from build123d import *

# Parameters (mm, degrees)
BOSS_EXTRUDE1_DEPTH                                 = 15
M24X2_0_TAPPED_HOLE1_D                              = 22
M24X2_0_TAPPED_HOLE1_DEPTH                          = 58
M24X2_0_TAPPED_HOLE1_TIP                            = 6.609466809
CBORE_FOR_M5_HEX_SOCKET_HEAD_CAP_SCREW1_D           = 5.5
CBORE_FOR_M5_HEX_SOCKET_HEAD_CAP_SCREW1_CBORE_D     = 8.5
CBORE_FOR_M5_HEX_SOCKET_HEAD_CAP_SCREW1_CBORE_DEPTH = 5
CIRPATTERN3_COUNT                                   = 6


with BuildPart() as part:
    # Sketch1 → Boss-Extrude1 (new body)
    with BuildSketch(Plane.XY):
        with BuildLine():
            Line((-2.5, 29), (2.5, 29))
            Line((2.5, 29), (2.991048754, 29.850521392))
            ThreePointArc((2.991048754, 29.850521392), (9.270509831, 28.531695489), (15.125886974, 25.907673443))
            Line((15.125886974, 25.907673443), (15.023229831, 24.930955968))
            Line((15.023229831, 24.930955968), (19.068314802, 21.992029706))
            Line((19.068314802, 21.992029706), (19.965505521, 22.39148475))
            ThreePointArc((19.965505521, 22.39148475), (24.270509831, 17.633557569), (27.465247988, 12.068974809))
            Line((27.465247988, 12.068974809), (26.808096487, 11.339134128))
            Line((26.808096487, 11.339134128), (28.353181458, 6.583851546))
            Line((28.353181458, 6.583851546), (29.31381778, 6.379661993))
            ThreePointArc((29.31381778, 6.379661993), (30, 0), (29.31381778, -6.379661993))
            Line((29.31381778, -6.379661993), (28.353181458, -6.583851546))
            Line((28.353181458, -6.583851546), (26.808096487, -11.339134128))
            Line((26.808096487, -11.339134128), (27.465247988, -12.068974809))
            ThreePointArc((27.465247988, -12.068974809), (24.270509831, -17.633557569), (19.965505521, -22.39148475))
            Line((19.965505521, -22.39148475), (19.068314802, -21.992029706))
            Line((19.068314802, -21.992029706), (15.023229831, -24.930955968))
            Line((15.023229831, -24.930955968), (15.125886974, -25.907673443))
            ThreePointArc((15.125886974, -25.907673443), (9.270509831, -28.531695489), (2.991048754, -29.850521392))
            Line((2.991048754, -29.850521392), (2.5, -29))
            Line((2.5, -29), (-2.5, -29))
            Line((-2.5, -29), (-2.991048754, -29.850521392))
            ThreePointArc((-2.991048754, -29.850521392), (-9.270509831, -28.531695489), (-15.125886974, -25.907673443))
            Line((-15.125886974, -25.907673443), (-15.023229831, -24.930955968))
            Line((-15.023229831, -24.930955968), (-19.068314802, -21.992029706))
            Line((-19.068314802, -21.992029706), (-19.965505521, -22.39148475))
            ThreePointArc((-19.965505521, -22.39148475), (-24.270509831, -17.633557569), (-27.465247988, -12.068974809))
            Line((-27.465247988, -12.068974809), (-26.808096487, -11.339134128))
            Line((-26.808096487, -11.339134128), (-28.353181458, -6.583851546))
            Line((-28.353181458, -6.583851546), (-29.31381778, -6.379661993))
            ThreePointArc((-29.31381778, -6.379661993), (-30, 0), (-29.31381778, 6.379661993))
            Line((-29.31381778, 6.379661993), (-28.353181458, 6.583851546))
            Line((-28.353181458, 6.583851546), (-26.808096487, 11.339134128))
            Line((-26.808096487, 11.339134128), (-27.465247988, 12.068974809))
            ThreePointArc((-27.465247988, 12.068974809), (-24.270509831, 17.633557569), (-19.965505521, 22.39148475))
            Line((-19.965505521, 22.39148475), (-19.068314802, 21.992029706))
            Line((-19.068314802, 21.992029706), (-15.023229831, 24.930955968))
            Line((-15.023229831, 24.930955968), (-15.125886974, 25.907673443))
            ThreePointArc((-15.125886974, 25.907673443), (-9.270509831, 28.531695489), (-2.991048754, 29.850521392))
            Line((-2.991048754, 29.850521392), (-2.5, 29))
        make_face()
    extrude(amount=BOSS_EXTRUDE1_DEPTH)

    # M24x2.0 Tapped Hole1
    with Locations(Plane.XY.offset(15)):
        with Locations((0, 0)):
            Hole(M24X2_0_TAPPED_HOLE1_D / 2, depth=M24X2_0_TAPPED_HOLE1_DEPTH)
            with Locations((0, 0, -(M24X2_0_TAPPED_HOLE1_DEPTH + M24X2_0_TAPPED_HOLE1_TIP / 2))):  # 118° drill point
                Cone(0, M24X2_0_TAPPED_HOLE1_D / 2, M24X2_0_TAPPED_HOLE1_TIP, mode=Mode.SUBTRACT)

    # CBORE for M5 Hex Socket Head Cap Screw1 (through all)
    with Locations(Plane.XY.offset(15)):
        with Locations((0, 19)):
            cbore_for_m5_hex_socket_head_cap_screw1 = CounterBoreHole(CBORE_FOR_M5_HEX_SOCKET_HEAD_CAP_SCREW1_D / 2, CBORE_FOR_M5_HEX_SOCKET_HEAD_CAP_SCREW1_CBORE_D / 2, CBORE_FOR_M5_HEX_SOCKET_HEAD_CAP_SCREW1_CBORE_DEPTH)

    # CirPattern3: CBORE for M5 Hex Socket Head Cap Screw1 ×6 about axis
    cirpattern3_axis = Axis((0, 0, 0), (0, 0, 1))
    for i in range(1, CIRPATTERN3_COUNT):
        add(cbore_for_m5_hex_socket_head_cap_screw1.rotate(cirpattern3_axis, i * 360 / CIRPATTERN3_COUNT), mode=Mode.SUBTRACT)


solid = part.part
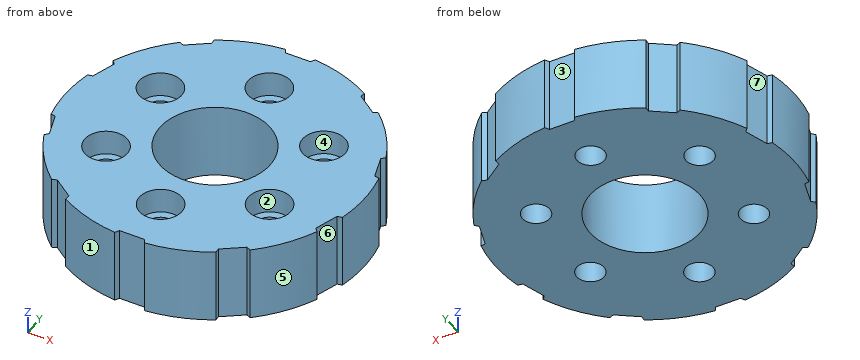
Could you check a few things on this model? Use its own coordinates, in mm. Face numbers are marked on the shaded views. A direction names the side the tool comes from. Coordinates: 2 decimals unless noted, no trailing zeros. Loops run counter-clockwise (first coordinate to the right, second up) from the corner with the lowest first, then second, coordinate; pieces in that order, holes last.
1. We'd pull the mould along Y, two halves only. Please class the marked faces 1, 2 and 3: released by +Y, released by -Y, zero draft, split by the parting line, or undercut.
2. Imagine slicing it at D-D (z = 8.5). Give the number of separate pieces and of enclosed holes in the cut face, and give its area (3 significant figures).
3. Imagine slicing it at C-C (y = -9.5). Please give me the cut outline in (x, z), and give its area (3 significant figures).
4. For the marked faces 4, 5, 6 and 7, which set-ups out of +Z, -Z, +X, -X, +Y, -Y let a thin tool reach every point of the face, with its end or its side?
5. Imagine slicing it at A-A (y = 0). Please give me the cut outline in (x, z), and give its area (3 significant figures).
6. I need wall thicknesses on L1, parallel to Y at x = 0, z = 8; L2, parallel to Y at x = -3, z = 11.5; L3, parallel to X at y = 12, z = 8. Which ranges of each line are inside material? Lowest first, please.
7. For P1, Ø1, axis at x = -10.5, z = 1.5, coming from the +Y side; P2, Ø4, axis at x = -18, y = -9.5, coming from the +Z side; P3, Ø1.5, axis at x = 0.5, z = 7, coming from the -Y side, each with a flat end and sliding along its axis, tell me the tip position at first contact or that it passes through.
8. Imagine slicing it at B-B (x = 6.5). Please give me the cut outline in (y, z).
Computed values:
1. face 1: released by -Y
1. face 2: undercut
1. face 3: released by +Y
2. separate pieces: 1
2. enclosed holes: 7
2. area: 2,250 mm2
3. outline: (-27.41, 0) - (-19.2, 0) - (-19.2, 10) - (-20.7, 10) - (-20.7, 15) - (-27.41, 15) - close; (-13.7, 0) - (-5.55, 0) - (-5.55, 15) - (-12.2, 15) - (-12.2, 10) - (-13.7, 10) - close; (5.55, 0) - (13.7, 0) - (13.7, 10) - (12.2, 10) - (12.2, 15) - (5.55, 15) - close; (19.2, 0) - (27.41, 0) - (27.41, 15) - (20.7, 15) - (20.7, 10) - (19.2, 10) - close
3. area: 461 mm2
4. face 4: +Z
4. face 5: +Z, -Z, +X, -Y
4. face 6: +Z, -Z, +X
4. face 7: +Z, -Z, -X
5. outline: (-30, 0) - (-11, 0) - (-11, 15) - (-30, 15) - close; (11, 0) - (30, 0) - (30, 15) - (11, 15) - close
5. area: 570 mm2
6. L1: y = -29 to -21.75, -16.25 to -11, 11 to 16.25, 21.75 to 29
6. L2: y = -29.85 to -22.01, -15.99 to -10.58, 10.58 to 15.99, 22.01 to 29.85
6. L3: x = -27.4 to -17.6, -15.31 to 15.31, 17.6 to 27.4
7. P1: stops at y = 28.28
7. P2: stops at z = 10
7. P3: stops at y = -29
8. outline: (-29.29, 0) - (-8.87, 0) - (-8.87, 15) - (-29.29, 15) - close; (8.87, 0) - (29.29, 0) - (29.29, 15) - (8.87, 15) - close
